The model under review builds one solid part; all positions refer to its coordinate system, in mm. Round coordinates to 2 decimals unless told otherwise and drop trailing zeros. Order: outer loops, then holes, each group sorted by start corner. A loop starts at its lowest first (then second) coordinate and runs counter-clockwise, first axis right, second up. Notation, with made-up numbers: M 81.25,68.25 L 109.25,68.25 A23 cw 109.25,96.25 Z; hole C 76.5,39 d11. An arc over 180 degrees is marked long. Use a Markdown table: item, result. Add a question column.
1. Insertion check: P1, Ø21, axis at x = 123.317, z = 147.828, coming from the -Y side; P2, Ø1.4, axis at y = -2, z = 51, coming from the +X side; P3, Ø18, axis at x = 58.13, z = 118.28, coming from the +Y side. Each pin has a flat end and moves straight along its axis. Give the tip position at first contact, or say it passes through.
2. Consider section D-D on x = 154. State the section outline as (y, z) points.
3. Consider section B-B on x = 23.5. State the section outline as (y, z) points, then the cut area to 3 significant figures.
4. The part is to be moulded in two halves that separate along Z. For faces 1 (the cylindrical face through (130.95, -2.35, 150.23)), 2 (the cylindrical face through (9.607, -2.348, 27.64)), 3 (the flat face through (20.6, -2.3, 150.1)), 4 (the flat face through (99, -4.762, 157)), say which applies: +Z half, -Z half, draft (parallel to the pull), parting line (faces both ways), or undercut.
5. To check wall thickness, follow probe 1 along X at (y, z) = (-3.9, 80); probe 2 along X at (y, z) = (-2.3, 15); probe 3 along Z at (x, y) = (241, -2.8) (3 decimals). State the ranges of each line that lie inside material, in increasing order.
6. Consider section C-C on y = -2.6. Count the separate pieces of the cut face and the enclosed holes in it, then the cut area to 3 significant figures.
7. Consider section A-A on z = 152. State the section outline as (x, y) points.
from build123d import *

# Parameters (mm, degrees)
F0_R     = 19.177
F0_R_2   = 11.1125
F0_R_3   = 8.001
F1_DEPTH = 4.7625


with BuildPart() as f1:
    # F0 (on Front) → F1 (new body)
    with BuildSketch(Plane.XZ):
        with BuildLine():
            ThreePointArc((0, 8.382), (2.455031, 2.455031), (8.382, 0))
            Line((8.382, 0), (105.918, 0))
            ThreePointArc((105.918, 0), (111.844969, 2.455031), (114.3, 8.382))
            Line((114.3, 8.382), (114.3, 80.645))
            ThreePointArc((114.3, 80.645), (129.178976, 116.566024), (165.1, 131.445))
            Line((165.1, 131.445), (243.967, 131.445))
            ThreePointArc((243.967, 131.445), (255.55153, 136.24347), (260.35, 147.828))
            Line((260.35, 147.828), (260.35, 220.853))
            ThreePointArc((260.35, 220.853), (257.013104, 230.762685), (248.361737, 236.635553))
            Line((248.361737, 236.635553), (188.275211, 253.36697))
            ThreePointArc((188.275211, 253.36697), (185.980128, 253.841011), (183.642, 254))
            ThreePointArc((183.642, 254), (181.19937, 253.826408), (178.80584, 253.30912))
            Line((178.80584, 253.30912), (118.94312, 235.84916))
            ThreePointArc((118.94312, 235.84916), (118.094256, 235.575044), (117.262422, 235.252921))
            Line((117.262422, 235.252921), (50.745696, 207.285359))
            ThreePointArc((50.745696, 207.285359), (44.679286, 203.216493), (40.588503, 197.16484))
            Line((40.588503, 197.16484), (0, 101.6))
            Line((0, 101.6), (0, 8.382))
        make_face()
        with Locations((28.7655, 26.797)):
            Circle(F0_R, mode=Mode.SUBTRACT)
        with Locations((87.503, 26.797)):
            Circle(F0_R, mode=Mode.SUBTRACT)
        with Locations((28.7655, 81.026)):
            Circle(F0_R, mode=Mode.SUBTRACT)
        with Locations((58.13425, 118.275273)):
            Circle(F0_R_2, mode=Mode.SUBTRACT)
        with Locations((87.503, 81.026)):
            Circle(F0_R, mode=Mode.SUBTRACT)
        with Locations((58.13425, 189.712773)):
            Circle(F0_R_2, mode=Mode.SUBTRACT)
        with Locations((123.317, 147.828)):
            Circle(F0_R_3, mode=Mode.SUBTRACT)
        with Locations((123.317, 220.853)):
            Circle(F0_R_3, mode=Mode.SUBTRACT)
        with Locations((183.642, 147.828)):
            Circle(F0_R_3, mode=Mode.SUBTRACT)
        with Locations((243.967, 147.828)):
            Circle(F0_R_3, mode=Mode.SUBTRACT)
        with Locations((183.642, 236.728)):
            Circle(F0_R_3, mode=Mode.SUBTRACT)
        with Locations((243.967, 220.853)):
            Circle(F0_R_3, mode=Mode.SUBTRACT)
    extrude(amount=F1_DEPTH)


solid = f1.part
Answer block:
| question | item | result |
|---|---|---|
| 1 | P1 | y = -4.76 |
| 1 | P2 | x = 114.3 |
| 1 | P3 | through |
| 2 | outline | M -4.76,130.22 L 0,130.22 L 0,246.07 L -4.76,246.07 Z |
| 3 | outline | M -4.76,0 L 0,0 L 0,8.36 L -4.76,8.36 Z; M -4.76,45.24 L 0,45.24 L 0,62.59 L -4.76,62.59 Z; M -4.76,99.47 L 0,99.47 L 0,156.93 L -4.76,156.93 Z |
| 3 | area | 396 mm^2 |
| 4 | face 1 | undercut |
| 4 | face 2 | undercut |
| 4 | face 3 | +Z half |
| 4 | face 4 | draft |
| 5 | probe 1 | 0 to 9.62, 47.92 to 68.35, 106.65 to 114.3 |
| 5 | probe 2 | 0 to 13.65, 43.88 to 72.38, 102.62 to 114.3 |
| 5 | probe 3 | 131.445 to 140.397, 155.259 to 213.422, 228.284 to 238.685 |
| 6 | separate pieces | 1 |
| 6 | enclosed holes | 12 |
| 6 | area | 32,500 mm^2 |
| 7 | outline | M 21.41,-4.76 L 116.49,-4.76 L 116.49,0 L 21.41,0 Z; M 130.14,-4.76 L 176.81,-4.76 L 176.81,0 L 130.14,0 Z; M 190.47,-4.76 L 237.14,-4.76 L 237.14,0 L 190.47,0 Z; M 250.79,-4.76 L 260.35,-4.76 L 260.35,0 L 250.79,0 Z |
